from build123d import *

# Parameters (mm, degrees)
F0_R     = 4
F1_DEPTH = 4
F0_R_2   = 11
F2_DEPTH = 2


with BuildPart() as f1:
    # F0 (on Top) → F1 (new body, symmetric)
    with BuildSketch(Plane.XY):
        Circle(F0_R)
        with BuildLine():
            ThreePointArc((-2.304886, -1.5), (-2.75, 0), (-2.304886, 1.5))
            Line((-2.304886, 1.5), (2.304886, 1.5))
            ThreePointArc((2.304886, 1.5), (2.75, 0), (2.304886, -1.5))
            Line((2.304886, -1.5), (-2.304886, -1.5))
        make_face(mode=Mode.SUBTRACT)
    extrude(amount=F1_DEPTH, both=True)

    # F0 (on Top) → F2 (join)
    with BuildSketch(Plane.XY):
        Circle(F0_R_2)
        with BuildLine():
            Line((-8.314696, -5.555702), (-5.946591, -3.973385))
            ThreePointArc((-5.946591, -3.973385), (-5.545353, -4.552303), (-5.087967, -5.087967))
            Line((-5.087967, -5.087967), (-7.071068, -7.071068))
            ThreePointArc((-7.071068, -7.071068), (-7.730105, -6.343933), (-8.314696, -5.555702))
        make_face(mode=Mode.SUBTRACT)
        with BuildLine():
            ThreePointArc((0, -10), (-0.980171, -9.951847), (-1.950903, -9.807853))
            Line((-1.950903, -9.807853), (-1.419245, -7.135026))
            ThreePointArc((-1.419245, -7.135026), (-0.713336, -7.24397), (0, -7.280411))
            Line((0, -7.280411), (0, -10))
        make_face(mode=Mode.SUBTRACT)
        with BuildLine():
            Line((-5.555702, -8.314696), (-4.017561, -6.012706))
            ThreePointArc((-4.017561, -6.012706), (-3.41521, -6.390758), (-2.77761, -6.705743))
            Line((-2.77761, -6.705743), (-3.826834, -9.238795))
            ThreePointArc((-3.826834, -9.238795), (-4.713967, -8.819213), (-5.555702, -8.314696))
        make_face(mode=Mode.SUBTRACT)
        with BuildLine():
            Line((-9.807853, -1.950903), (-6.91385, -1.37525))
            ThreePointArc((-6.91385, -1.37525), (-6.771225, -2.055379), (-6.561866, -2.718014))
            Line((-6.561866, -2.718014), (-9.238795, -3.826834))
            ThreePointArc((-9.238795, -3.826834), (-9.569403, -2.902847), (-9.807853, -1.950903))
        make_face(mode=Mode.SUBTRACT)
        with BuildLine():
            Line((1.950903, -9.807853), (1.419245, -7.135026))
            ThreePointArc((1.419245, -7.135026), (2.109376, -6.95503), (2.77761, -6.705743))
            Line((2.77761, -6.705743), (3.826834, -9.238795))
            ThreePointArc((3.826834, -9.238795), (2.902847, -9.569403), (1.950903, -9.807853))
        make_face(mode=Mode.SUBTRACT)
        with BuildLine():
            Line((5.555702, -8.314696), (4.017561, -6.012706))
            ThreePointArc((4.017561, -6.012706), (4.576183, -5.577444), (5.087967, -5.087967))
            Line((5.087967, -5.087967), (7.071068, -7.071068))
            ThreePointArc((7.071068, -7.071068), (6.343933, -7.730105), (5.555702, -8.314696))
        make_face(mode=Mode.SUBTRACT)
        with BuildLine():
            Line((8.314696, -5.555702), (5.946591, -3.973385))
            ThreePointArc((5.946591, -3.973385), (6.285648, -3.361098), (6.561866, -2.718014))
            Line((6.561866, -2.718014), (9.238795, -3.826834))
            ThreePointArc((9.238795, -3.826834), (8.819213, -4.713967), (8.314696, -5.555702))
        make_face(mode=Mode.SUBTRACT)
        with BuildLine():
            Line((9.807853, -1.950903), (6.91385, -1.37525))
            ThreePointArc((6.91385, -1.37525), (6.988029, -0.689611), (6.994381, 0))
            Line((6.994381, 0), (10, 0))
            ThreePointArc((10, 0), (9.951847, -0.980171), (9.807853, -1.950903))
        make_face(mode=Mode.SUBTRACT)
        with BuildLine():
            Line((-9.807853, 1.950903), (-6.806542, 1.353905))
            ThreePointArc((-6.806542, 1.353905), (-6.933587, 0.681549), (-6.994381, 0))
            Line((-6.994381, 0), (-10, 0))
            ThreePointArc((-10, 0), (-9.951847, 0.980171), (-9.807853, 1.950903))
        make_face(mode=Mode.SUBTRACT)
        with BuildLine():
            Line((-8.314696, 5.555702), (-5.687525, 3.800283))
            ThreePointArc((-5.687525, 3.800283), (-6.053617, 3.234376), (-6.363586, 2.635884))
            Line((-6.363586, 2.635884), (-9.238795, 3.826834))
            ThreePointArc((-9.238795, 3.826834), (-8.819213, 4.713967), (-8.314696, 5.555702))
        make_face(mode=Mode.SUBTRACT)
        with BuildLine():
            Line((-5.555702, 8.314696), (-3.758495, 5.624986))
            ThreePointArc((-3.758495, 5.624986), (-4.302483, 5.241241), (-4.807556, 4.807556))
            Line((-4.807556, 4.807556), (-7.071068, 7.071068))
            ThreePointArc((-7.071068, 7.071068), (-6.343933, 7.730105), (-5.555702, 8.314696))
        make_face(mode=Mode.SUBTRACT)
        with BuildLine():
            Line((-1.950903, 9.807853), (-1.311936, 6.595549))
            ThreePointArc((-1.311936, 6.595549), (-1.954337, 6.441238), (-2.579329, 6.227051))
            Line((-2.579329, 6.227051), (-3.826834, 9.238795))
            ThreePointArc((-3.826834, 9.238795), (-2.902847, 9.569403), (-1.950903, 9.807853))
        make_face(mode=Mode.SUBTRACT)
        Circle(F0_R, mode=Mode.SUBTRACT)
        with BuildLine():
            Line((9.807853, 1.950903), (6.806542, 1.353905))
            ThreePointArc((6.806542, 1.353905), (6.616187, 2.005648), (6.363586, 2.635884))
            Line((6.363586, 2.635884), (9.238795, 3.826834))
            ThreePointArc((9.238795, 3.826834), (9.569403, 2.902847), (9.807853, 1.950903))
        make_face(mode=Mode.SUBTRACT)
        with BuildLine():
            Line((8.314696, 5.555702), (5.687525, 3.800283))
            ThreePointArc((5.687525, 3.800283), (5.271653, 4.324985), (4.807556, 4.807556))
            Line((4.807556, 4.807556), (7.071068, 7.071068))
            ThreePointArc((7.071068, 7.071068), (7.730105, 6.343933), (8.314696, 5.555702))
        make_face(mode=Mode.SUBTRACT)
        with BuildLine():
            Line((5.555702, 8.314696), (3.758495, 5.624986))
            ThreePointArc((3.758495, 5.624986), (3.183178, 5.953959), (2.579329, 6.227051))
            Line((2.579329, 6.227051), (3.826834, 9.238795))
            ThreePointArc((3.826834, 9.238795), (4.713967, 8.819213), (5.555702, 8.314696))
        make_face(mode=Mode.SUBTRACT)
        with BuildLine():
            Line((1.950903, 9.807853), (1.311936, 6.595549))
            ThreePointArc((1.311936, 6.595549), (0.658893, 6.68851), (0, 6.719589))
            Line((0, 6.719589), (0, 10))
            ThreePointArc((0, 10), (0.980171, 9.951847), (1.950903, 9.807853))
        make_face(mode=Mode.SUBTRACT)
    extrude(amount=F2_DEPTH)


solid = f1.part
Read the model definition and answer for the solid it produces. Units are mm, in the model's axes. Round coordinates to 2 decimals unless told otherwise and drop trailing zeros. Write each loop counter-clockwise with the first axis right and the second up, starting at its lowest first coordinate (ties: lowest second). Pieces come first, ordered by that corner, then holes. Notation, with made-up numbers: M 80,57 L 135,57 A13 cw 135,81 Z; hole C -30,-26 d10. An arc over 180 degrees is marked long. Use a Markdown table: item, result.
1) The part is cut by section C-C (x = 0.75). Write down the section's boundary in (y, z), plus the area to 3 significant figures.
Answers follow:
| item | result |
|---|---|
| outline | M -10.97,0 L -3.93,0 L -3.93,-4 L -1.5,-4 L -1.5,4 L -3.93,4 L -3.93,2 L -10.97,2 Z; M 1.5,-4 L 3.93,-4 L 3.93,0 L 6.68,0 L 6.68,2 L 3.93,2 L 3.93,4 L 1.5,4 Z; M 9.97,0 L 10.97,0 L 10.97,2 L 9.97,2 Z |
| area | 60.5 mm2 |
2) Straight lines are drawn through the part: line 1 along Y through (x, z) = (-6.25, 1.75); line 2 along X through (y, z) = (0.5, 0.25); line 3 along Y through (x, z) = (4.25, 0.5). For each, find the intervals that lie inside material, in ascending order. Write a range as [from, to].
Answers follow:
| item | result |
|---|---|
| line 1 | y = [-9.05, -6.25], [-4.18, 2.87], [4.18, 6.25], [7.81, 9.05] |
| line 2 | x = [-10.99, -9.99], [-6.96, -2.7], [2.7, 10.99] |
| line 3 | y = [-10.15, -6.36], [-5.84, 6.36], [9.05, 10.15] |
3) For a pull along Y with two mould halves and no side action, classify faces 1 (the cylindrical face through (8.826, -4.702, 0.986)), 2 (the flat face through (0, -2, -4)) as pulls with the +Y half, pulls with the -Y half, needs draft (parallel to the pull), parting line crosses it, or undercut.
Answers follow:
| item | result |
|---|---|
| face 1 | undercut |
| face 2 | needs draft |
4) The part is cut by section D-D (y = 8.75). Write down the section's boundary in (x, z), plus the area to 3 significant figures.
Answers follow:
| item | result |
|---|---|
| outline | M -6.67,0 L -3.62,0 L -3.62,2 L -6.67,2 Z; M -1.74,0 L 0,0 L 0,2 L -1.74,2 Z; M 1.74,0 L 3.62,0 L 3.62,2 L 1.74,2 Z; M 4.84,0 L 6.67,0 L 6.67,2 L 4.84,2 Z |
| area | 17.0 mm2 |
5) The part is cut by section A-A (x = 7.5). Write down the section's boundary in (y, z).
Answers follow:
| item | result |
|---|---|
| outline | M -8.05,0 L -5.01,0 L -5.01,2 L -8.05,2 Z; M -3.11,0 L -1.49,0 L -1.49,2 L -3.11,2 Z; M 0,0 L 1.49,0 L 1.49,2 L 0,2 Z; M 3.11,0 L 5.01,0 L 5.01,2 L 3.11,2 Z; M 6.61,0 L 8.05,0 L 8.05,2 L 6.61,2 Z |
6) The part is cut by section B-B (z = 3). Write down the section's boundary in (x, y), plus the area to 3 significant figures.
Answers follow:
| item | result |
|---|---|
| outline | C 0,0 d8; hole M -2.3,-1.5 L 2.3,-1.5 A2.75 ccw 2.3,1.5 L -2.3,1.5 A2.75 ccw Z |
| area | 34.6 mm2 |
7) Flat-ended cylindrical pins translate along their axes: pin 1 (1.4 mm diameter, centred on x = -1, z = -0.5, fed in from -Y); pin 2 (10 mm diameter, centred on x = 3, y = 4.5, fed in from +Z); pin 3 (0.6 mm diameter, centred on y = 8, z = 1.5, fed in from +X); pin 4 (2 mm diameter, centred on x = 4.5, y = 8, fed in from +Z). Find the tip coordinate at first contact, or state that the pin passes through.
Answers follow:
| item | result |
|---|---|
| pin 1 | stops at y = -10.99 |
| pin 2 | stops at z = 4 |
| pin 3 | stops at x = 7.86 |
| pin 4 | stops at z = 2 |
